from build123d import *

# Parameters (mm, degrees)
F0_R     = 14.25
F1_DEPTH = 41.5


# Not quite as in the source:
# - ends of sketch curves that miss each other by under 0.0002 mm in the source are joined


with BuildPart() as f1:
    # F0 (on Top) → F1 (new body, symmetric)
    with BuildSketch(Plane.XY):
        with BuildLine():
            ThreePointArc((-11.0000361821, 11.6189157839), (-4.98249e-05, 15.9999999999), (10.9999638179, 11.6189842932))
            Line((10.9999638179, 11.6189842932), (10.9999638179, 76.6189842932))
            ThreePointArc((10.9999638179, 76.6189842932), (3.42546e-05, 65.6189519658), (-10.9999638181, 76.6189157839))
            Line((-10.9999638181, 76.6189157839), (-11.0000361821, 11.6189157839))
        make_face()
        with BuildLine():
            ThreePointArc((-11.0000361821, 11.6189157839), (-6.3245324367, -14.6969483042), (16, 0))
            ThreePointArc((16, 0), (14.6969286092, 6.3245782039), (10.9999638179, 11.6189842932))
            ThreePointArc((10.9999638179, 11.6189842932), (-4.98249e-05, 15.9999999999), (-11.0000361821, 11.6189157839))
        make_face()
        Circle(F0_R, mode=Mode.SUBTRACT)
    extrude(amount=F1_DEPTH, both=True)


solid = f1.part
Could you check a few things on this model? Use its own coordinates, in mm. A direction names the side the tool comes from. Coordinates: 2 decimals unless noted, no trailing zeros. Write each loop counter-clockwise with the first axis right and the second up, starting at its lowest first coordinate (ties: lowest second). Pieces come first, ordered by that corner, then holes. Notation, with made-up numbers: M 27,43.5 L 64,43.5 A29 ccw 64,69.5 Z; hole C -25,-39.5 d9. An arc over 180 degrees is marked long. One line per question, with ' | ' between items.
1) Imagine slicing it at B-B, the plane z = -34. Write out the boundary of the cut face in (x, y), and give its area (3 significant figures).
Checks:
outline: M -11,11.62 A16 ccw long 11,11.62 L 11,76.62 A11 cw -11,76.62 Z; hole C 0,0 d28.5 | area: 1,340 mm²
2) If we mould it in two halves opening along Y, with no side actions, what happens to faces 3 (the face through (0.24, 65.62, 0.58)), 4 (the face through (13.163, -5.458, -0.581)), 5 (the face through (0, 41, -41.5))? For each: released by +Y, released by -Y, zero draft, split by the parting line, or undercut.
Checks:
face 3: released by +Y | face 4: undercut | face 5: zero draft
3) I need wall thicknesses on probe 1 along Y at (x, z) = (0, 10); probe 2 along Y at (x, z) = (6, 35.5); probe 3 along X at (y, z) = (12, -35.5). Which ranges of each line are inside material? Lowest first, please. Write a range as [from, to].
Checks:
probe 1: [-16, -14.25], [14.25, 65.62] | probe 2: [-14.83, -12.93], [12.93, 67.4] | probe 3: [-11, -7.69], [7.69, 11]
4) Imagine slicing it at A-A, the plane x = 0. Write out the boundary of the cut face in (y, z), and give its area (3 significant figures).
Checks:
outline: M -16,-41.5 L -14.25,-41.5 L -14.25,41.5 L -16,41.5 Z; M 14.25,-41.5 L 65.62,-41.5 L 65.62,41.5 L 14.25,41.5 Z | area: 4,410 mm²
5) For faces 1 (the face through (0, 41, 41.5)), 2 (the face through (11, 44, 1)), which set-ups out of +Z, -Z, +X, -X, +Y, -Y let a thin tool reach every point of the face, with its end or its side?
Checks:
face 1: +Z, +X, -X, +Y, -Y | face 2: +Z, -Z, +X, +Y
6) Imagine slicing it at D-D, the plane y = 53. Write out the boundary of the cut face in (x, z), and give its area (3 significant figures).
Checks:
outline: M -11,-41.5 L 11,-41.5 L 11,41.5 L -11,41.5 Z | area: 1,830 mm²
7) For pin 1 Ø19.5 at (y, z) = (31, 15) entering from -X; pin 2 Ø3 at (y, z) = (-1.5, -30) entering from +X; pin 3 Ø2 at (x, z) = (-3, 12) entering from +Y; pin 4 Ø6 at (x, z) = (-12.5, 0.5) entering from -Y, each with a flat end and sliding along its axis, tell me the tip position at first contact or that it passes through.
Checks:
pin 1: x = -11 | pin 2: x = 16 | pin 3: y = 66.37 | pin 4: y = -12.87
8) Imagine slicing it at C-C, the plane y = 69. Write out the boundary of the cut face in (x, z), and give its area (3 significant figures).
Checks:
outline: M -11,-41.5 L -7.93,-41.5 L -7.93,41.5 L -11,41.5 Z; M 7.93,-41.5 L 11,-41.5 L 11,41.5 L 7.93,41.5 Z | area: 509 mm²
